```python
from build123d import *


with BuildPart() as f1:
    # F0 (on Front) → F1 (revolve)
    with BuildSketch(Plane.XZ):
        Polygon((20, 35), (0, 35), (0, 5), (13.305354, 5), (20, 5), (24.382994, 5), (40, 5), (60, 5), (60, 15), (40, 15), (40, 25), (20, 25), align=None)
    revolve(axis=Axis((22.793579, 0, 0), (1, 0, 0)))

    # F2: F1 across plane


with BuildPart() as f1_1:
    add(f1.part)
    add(f1.part.mirror(Plane.YZ))


solid = f1_1.part
```
Model file for the job. Use its own axes, mm. A direction names the side the tool comes from. Coordinates: 2 decimals unless noted, no trailing zeros. Write each loop counter-clockwise with the first axis right and the second up, starting at its lowest first coordinate (ties: lowest second). Pieces come first, ordered by that corner, then holes. Notation, with made-up numbers: (65, 44.25) - (90, 44.25) arc R20 cw to (90, 64.25) - close; hole circle Ø8 at (81, 53.5). An arc over 180 degrees is marked (long way). One line per item, written item: value. Start each with the question number.
1. Slice it at D-D (z = -7.5). Write the cut outline in (x, y).
2. Probe line 1 (Y direction, x = 46, z = 0); line 2 (Z direction, x = -33, y = 0); line 3 (Y direction, x = -9, z = 0). List the from-to ranges inside material, lowest first. Write a range as from..to.
3. Tool access for faces 4 (the flat face through (40, 11, -11)), 5 (the flat face through (60, -4, 4)), 6 (the cylindrical face through (-29.86, -7.509, 23.846)): list every direction of +Z, -Z, +X, -X, +Y, -Y with a clear straight run to the whole face (end or side of a thin tool).
4. Slice it at C-C (x = -27). Write the cut outline in (y, z), plus the area to 3 significant figures.
5. Mould opens along Y. For faces 1 (the cylindrical face through (0.84, 4.88, -1.08)), 2 (the cylindrical face through (-49.86, -0.66, -14.985)), 3 (the flat face through (-20, -8, 24)) say: released by +Y, released by -Y, zero draft, split by the parting line, or undercut.
6. Slice it at A-A (z = 0). Write the cut outline in (x, y).
7. Flat gauge pins, fed straight in: pin 1 (5 mm diameter, centred on x = 4.5, z = 5.5, fed in from -Y); pin 2 (1.5 mm diameter, centred on y = 16.5, z = -9, fed in from -X); pin 3 (8 mm diameter, centred on y = -3.5, z = 15, fed in from +X); pin 4 (12 mm diameter, centred on x = 18.5, z = -16.5, fed in from -Y). Where does each tip first touch, or does it go through?
Answers below:
1. outline: (-60, -12.99) - (-40, -12.99) - (-40, -23.85) - (-20, -23.85) - (-20, -34.19) - (20, -34.19) - (20, -23.85) - (40, -23.85) - (40, -12.99) - (60, -12.99) - (60, 12.99) - (40, 12.99) - (40, 23.85) - (20, 23.85) - (20, 34.19) - (-20, 34.19) - (-20, 23.85) - (-40, 23.85) - (-40, 12.99) - (-60, 12.99) - close
2. line 1: y = -15..-5, 5..15
2. line 2: z = -25..-5, 5..25
2. line 3: y = -35..-5, 5..35
3. face 4: +X
3. face 5: +Z, -Z, +X, +Y, -Y
3. face 6: -X
4. outline: circle Ø50 at (0, 0); hole circle Ø10 at (0, 0)
4. area: 1,880 mm^2
5. face 1: undercut
5. face 2: split by the parting line
5. face 3: zero draft
6. outline: (-60, -15) - (-40, -15) - (-40, -25) - (-20, -25) - (-20, -35) - (20, -35) - (20, -25) - (40, -25) - (40, -15) - (60, -15) - (60, -5) - (-60, -5) - close; (-60, 5) - (60, 5) - (60, 15) - (40, 15) - (40, 25) - (20, 25) - (20, 35) - (-20, 35) - (-20, 25) - (-40, 25) - (-40, 15) - (-60, 15) - close
7. pin 1: stops at y = -34.87
7. pin 2: stops at x = -40
7. pin 3: stops at x = 60
7. pin 4: stops at y = -33.39
